For this review, take the finished solid that the model builds, in its own axes (mm). Face numbers are marked on the shaded views. A direction names the side the tool comes from. Round coordinates to 2 decimals unless told otherwise and drop trailing zeros. Order: outer loops, then holes, each group sorted by start corner. A loop starts at its lowest first (then second) coordinate and runs counter-clockwise, first axis right, second up. Notation, with made-up numbers: (25, 82.5) -> (54, 82.5) arc R31 cw to (54, 118.5) -> close; hole circle Ø6 at (55, -40). An arc over 180 degrees is marked (long way). Use a Markdown table: item, result. Add a question column.
1) Consider section A-A (x = 2.5). State the section outline as (y, z) points.
2) Wall thickness on line 1 along X through (y, z) = (-1.25, 4); line 2 along Y through (x, z) = (-2.5, 1); line 3 along Z through (x, y) = (0.5, -1): over which ranges is each line inside the solid? List them lowest first. Write a range as [from, to].
3) Machinability: for the marked faces 1 and 2, which of the approach directions +Z, -Z, +X, -X, +Y, -Y give a long, thin tool a straight path to every point of the face, cutting with its end or side? Answer none if there is none.
4) Draft analysis for pull direction Z (two halves, no side actions). For the marked faces 3, 4, 5 and 6, state which applies: pulls with the +Z half, pulls with the -Z half, needs draft (parallel to the pull), parting line crosses it, or undercut.
5) Clearance check with flat-ended pins moving along their axes: P1, Ø6, axis at x = 11, z = 1, coming from the -Y side; P2, Ø4, axis at x = -2.5, y = -3.5, coming from the +Z side. State where each tip first meets the part, or that it passes through.
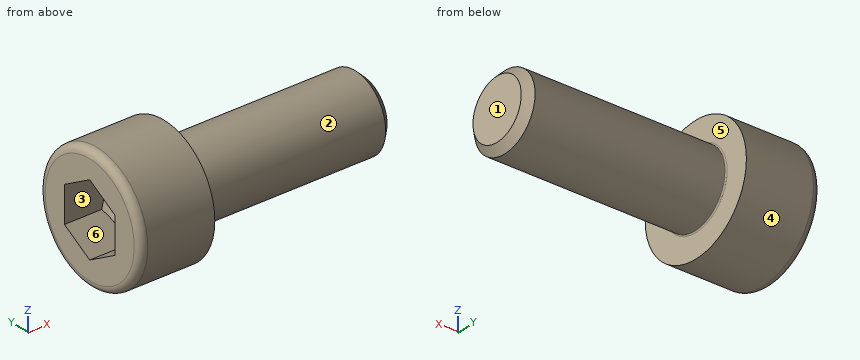
Autodesk Inventor part; units mm, degrees
ref_plane "Work Plane1" through (29, 0, 0) normal (0, -1, 0) x (1, 0, 0)
ref_plane "YZ Plane" through (0, 0, 0) normal (1, 0, 0) x (0, 1, 0)
ref_plane "XZ Plane" through (0, 0, 0) normal (0, 1, 0) x (-1, 0, 0)
sketch "Sketch1" plane through (0, 0, 0) normal (0, 0, 1) x (1, 0, 0)
  line L0 (-1.3333, 0) -> (16, 0)
  line L1 (16, 0) -> (16, 3)
  line L2 (16, 3) -> (3, 3)
  line L3 (3, 3) -> (2.3864, 3)
  line L4 (2.3864, 3) -> (0, 3)
  line L5 (0, 3) -> (0, 5)
  line L6 (0, 5) -> (-6, 5)
  line L7 (-6, 5) -> (-6, 2.8868)
  line L8 (-6, 2.8868) -> (-3, 2.8868)
  line L9 (-3, 2.8868) -> (-1.3333, 0)
  line L10 (-10.4, 0) -> (20.4, 0)
  line L11 (0, -1) -> (0, 6)
  line L12 (3, 3) -> (0, 3) construction
  dimension "d1" = 13
  dimension "d2" = 0.6136
  dimension "d3" = 6
  dimension "d4" = 3
  dimension "d5" = 60
  dimension "d6" = 6
  dimension "d7" = 6
  dimension "d8" = 5.7735
  dimension "d9" = 10
  dimension "d26" = 16
revolve "Body" add sketch "Sketch1" angle 360 about axis through (-1.3333, 0, 0) along (1, 0, 0)
sketch "Sketch2" plane through (-6, 0, 0) normal (-1, 0, 0) x (0, 0, 1)
  circle A0 centre (0, 0) radius 2.8868
  line L0 (0, -7) -> (0, 7)
  line L1 (-7, 0) -> (7, 0)
  line L2 (2.8868, 0) -> (1.4434, -2.5)
  line L3 (1.4434, -2.5) -> (-1.4434, -2.5)
  line L4 (-1.4434, -2.5) -> (-2.8868, 0)
  line L5 (-2.8868, 0) -> (-1.4434, 2.5)
  line L6 (-1.4434, 2.5) -> (1.4434, 2.5)
  line L7 (1.4434, 2.5) -> (2.8868, 0)
extrude "Slot" add sketch "Sketch2" against normal up to next contours L7 A0 | A0 L2 | L6 L0 A0 | A0 L0 L3 | L0 L6 A0 | A0 L3 L0 | L4 A0 | A0 L5
fillet "Fillet1" radius 0.6 1 edges at (-6, -5, 0)
thread "Thread"
chamfer "Chamfer1" distance 0.6135 distance2 0.6135 1 edges at (16, -3, 0) measured on face at (16, -1.1424, 0.935)
ref_plane "Work Plane1" through (29, 0, 0) normal (0, -1, 0) x (1, 0, 0)
fillet "Fillet2" radius 0.1 1 edges at (0, -3, 0)
equation "\"d30\" = R"
equation "\"d17\" = RR"
equation "\"d13\" = GEL"
equation "\"d15\" = -0.5 * SPD + 0.5 * GD"
equation "\"d16\" = GUL"
equation "\"d1\" = GEL"
equation "\"d3\" = KOH"
equation "\"d4\" = INTI"
equation "\"d6\" = GD"
equation "\"d7\" = BDM"
equation "\"d8\" = 1.1547 * SW"
equation "\"d9\" = KOD"
equation "\"d26\" = NLG"
equation "\"GD\" = NND"
equation "\"NLG\" = 16"
equation "\"GEL\" = 13"
equation "\"KOD\" = 10"
equation "\"KOH\" = 6"
equation "\"INTI\" = 3"
equation "\"GAL\" = 0.61345 * PTC"
equation "\"GUL\" = 0.61345 * PTC"
equation "\"BDM\" = NND"
equation "\"SW\" = 5"
equation "\"RR\" = 0.6"
equation "\"SPD\" = NND - 1.2269 * PTC"
equation "\"R\" = 0.1"
equation "\"PHH\" = 0.25"
equation "\"GD1\" = THREADDIA - 1.2269 * PTC"
equation "\"THREADDIA\" = 6"
equation "\"FAWI\" = 45deg"
equation "\"PTC\" = 1"
equation "\"NND\" = 6"
equation "\"TOA\" = 30deg"
equation "\"E0\" = 1.155 * SW"
properties part number "JIS B 1176 - M6 x 16" material "Steel, Mild"
Results list:
| question | item | result |
|---|---|---|
| 1 | outline | circle Ø6 at (0, 0) |
| 2 | line 1 | [-6, 0] |
| 2 | line 2 | [-4.9, -1.76], [1.76, 4.9] |
| 2 | line 3 | [-2.83, 2.83] |
| 3 | face 1 | +Z, -Z, +X, +Y, -Y |
| 3 | face 2 | +X |
| 4 | face 3 | undercut |
| 4 | face 4 | parting line crosses it |
| 4 | face 5 | needs draft |
| 4 | face 6 | undercut |
| 5 | P1 | y = -3 |
| 5 | P2 | z = 4.77 |
